from build123d import *

# Parameters (mm, degrees)
SKETCH1_W           = 90
SKETCH1_H           = 110
SKETCH1_R           = 3.25
SKETCH1_R_2         = 2.5
BOSS_EXTRUDE1_DEPTH = 3


with BuildPart() as part:
    # Sketch1 → Boss-Extrude1 (new body)
    with BuildSketch(Plane(origin=(0, 0, 0), x_dir=(1, 0, 0), z_dir=(0, 1, 0))):
        Rectangle(SKETCH1_W, SKETCH1_H)
        with Locations(Location((-30, 30, 0), (0, 0, 270))):
            Circle(SKETCH1_R, mode=Mode.SUBTRACT)
        with Locations(Location((-30, -30, 0), (0, 0, 270))):
            Circle(SKETCH1_R, mode=Mode.SUBTRACT)
        with Locations(Location((-5, 15, 0), (0, 0, 270))):
            Circle(SKETCH1_R_2, mode=Mode.SUBTRACT)
        with Locations(Location((35, 15, 0), (0, 0, 270))):
            Circle(SKETCH1_R_2, mode=Mode.SUBTRACT)
        with Locations(Location((35, -15, 0), (0, 0, 270))):
            Circle(SKETCH1_R_2, mode=Mode.SUBTRACT)
        with Locations(Location((-5, -15, 0), (0, 0, 270))):
            Circle(SKETCH1_R_2, mode=Mode.SUBTRACT)
        with Locations(Location((15, -40, 0), (0, 0, 270))):
            Circle(SKETCH1_R, mode=Mode.SUBTRACT)
        with Locations(Location((15, 40, 0), (0, 0, 270))):
            Circle(SKETCH1_R, mode=Mode.SUBTRACT)
    extrude(amount=BOSS_EXTRUDE1_DEPTH)


solid = part.part
Design review of the part built by this model. Coordinates are the model's own, in mm. Give positions to 0.01 mm unless a question says otherwise; leave off trailing zeros. Order: outer loops, then holes, each group sorted by start corner. A loop starts at its lowest first (then second) coordinate and runs counter-clockwise, first axis right, second up. Notation, with made-up numbers: (1, 31.5) - (15, 31.5) arc R7 cw to (15, 36.5) - close; hole circle Ø4 at (-18, -3). An arc over 180 degrees is marked (long way). Write item = value, one per line. Start each with the question number.
Q1. Clearance check with a flat-ended pin moving along its axis: pin 1 Ø4 at (x, z) = (35, -15) entering from +Y. State where the tip first meets the part, or that it passes through.
Q2. We need section C-C on z = -15. State the section outline as (x, y) points, plus the area to 3 significant figures.
Q3. To check wall thickness, follow L1, parallel to X at y = 1.5, z = 40; L2, parallel to Z at x = -28.5, y = 0.8; L3, parallel to Z at x = -32.5, y = 0.8. State the ranges of each line that lie inside material, in increasing order. Write a range as from..to.
Q4. We need section D-D on y = 0.9. State how many separate pieces and enclosed holes the cut face has, plus the area to 3 significant figures.
Q5. Mouldability with a two-part tool opening along Z and no side actions: class faces 1 (the face through (15.98, 1.48, 43.1)), 2 (the face through (-1, 1, -55)), 3 (the face through (-1, 1, 55)), 4 (the face through (-1, 0, -1)) as released by +Z, released by -Z, zero draft, split by the parting line, or undercut.
Q6. We need section B-B on x = -30. State the section outline as (y, z) points, plus the area to 3 significant figures.
Q7. We need section A-A on z = -40. State the section outline as (x, y) points.
Working result:
q1.pin_1 = through
q2.outline = (-45, 0) - (-7.5, 0) - (-7.5, 3) - (-45, 3) - close; (-2.5, 0) - (32.5, 0) - (32.5, 3) - (-2.5, 3) - close; (37.5, 0) - (45, 0) - (45, 3) - (37.5, 3) - close
q2.area = 240 mm²
q3.L1 = -45..11.75, 18.25..45
q3.L2 = -55..-32.88, -27.12..27.12, 32.88..55
q3.L3 = -55..-32.08, -27.92..27.92, 32.08..55
q4.separate_pieces = 1
q4.enclosed_holes = 8
q4.area = 9,690 mm²
q5.face_1 = undercut
q5.face_2 = released by -Z
q5.face_3 = released by +Z
q5.face_4 = zero draft
q6.outline = (0, -55) - (3, -55) - (3, -33.25) - (0, -33.25) - close; (0, -26.75) - (3, -26.75) - (3, 26.75) - (0, 26.75) - close; (0, 33.25) - (3, 33.25) - (3, 55) - (0, 55) - close
q6.area = 291 mm²
q7.outline = (-45, 0) - (11.75, 0) - (11.75, 3) - (-45, 3) - close; (18.25, 0) - (45, 0) - (45, 3) - (18.25, 3) - close
